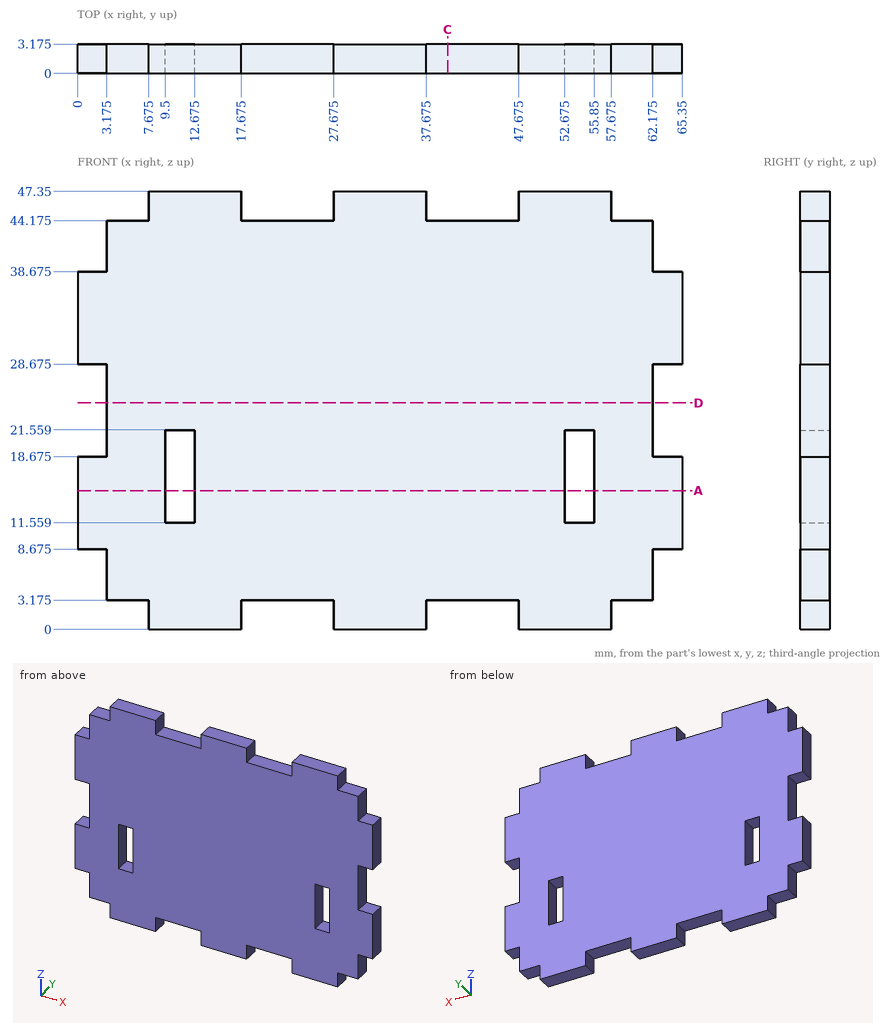
Geometry check sheet. Reference: drawing and pictorial views, mm from the part's lowest x, y, z. Give positions to 0.01 mm unless a question says otherwise; leave off trailing zeros. Order: outer loops, then holes, each group sorted by start corner. A loop starts at its lowest first (then second) coordinate and runs counter-clockwise, first axis right, second up. Notation, with made-up numbers: M 16,33.5 L 28,33.5 A30 cw 28,70.5 Z; hole C 2.25,41 d4. An arc over 180 degrees is marked long. Answer as a JSON object with one key per item and string values. Group by question number.
1) Cross-section at C-C (x = 40). Enter the section's corners in (y, z) (1 decimal).
2) Depth check by flat-ended pin: pin 1 Ø1.6 at (x, y) = (5.5, 1) entering from -Z (1 decimal); pin 2 Ø1.6 at (y, z) = (1.5, 1.5) entering from +X (1 decimal); pin 3 Ø1 at (y, z) = (1.5, 46) entering from -X (1 decimal). Enter the tip coordinate at first touch or a pass-through.
3) Cross-section at A-A (z = 15). Give the number of separate pieces and of enclosed holes in the cut face, then the cut area to 3 significant figures.
4) Scan lines: line 1 along X through (y, z) = (1, 44.5) (1 decimal); line 2 along Z through (x, y) = (3, 1.3) (1 decimal); line 3 along Z through (x, y) = (12.5, 1.55). Record each from-to range of solid material in increasing order. Write a range as [from, to].
5) Cross-section at D-D (z = 24.5). Enter the section's corners in (x, y) (1 decimal), then the cut area to 3 significant figures.
Result sheet:
{
 "1": {"outline": "M 0,3.2 L 3.2,3.2 L 3.2,44.2 L 0,44.2 Z"},
 "2": {"pin 1": "stops at z = 3.2", "pin 2": "stops at x = 57.7", "pin 3": "stops at x = 7.7"},
 "3": {"separate pieces": "3", "enclosed holes": "0", "area": "187 mm2"},
 "4": {"line 1": "x = [7.7, 17.7], [27.7, 37.7], [47.7, 57.7]", "line 2": "z = [8.7, 18.7], [28.7, 38.7]", "line 3": "z = [0, 11.56], [21.56, 47.35]"},
 "5": {"outline": "M 3.2,0 L 62.2,0 L 62.2,3.2 L 3.2,3.2 Z", "area": "187 mm2"}
}
